Design review of the part built by this model. Coordinates are the model's own, in mm. A direction names the side the tool comes from. Give positions to 0.01 mm unless a question says otherwise; leave off trailing zeros. Order: outer loops, then holes, each group sorted by start corner. A loop starts at its lowest first (then second) coordinate and runs counter-clockwise, first axis right, second up. Notation, with made-up numbers: (16, 38.25) -> (69, 38.25) arc R13 cw to (69, 58.25) -> close; hole circle Ø3 at (45.5, -4). An arc over 180 degrees is marked (long way). One line per item, written item: value.
Autodesk Inventor part; units mm, degrees
ref_plane "Work Plane1" through (0, 0, 0) normal (0, 0.7071068, -0.7071068) x (-1, 0, 0)
ref_plane "YZ Plane" through (0, 0, 0) normal (1, 0, 0) x (0, 1, 0)
sketch "Sketch1" plane through (0, 0, 0) normal (1, 0, 0) x (0, 1, 0)
  circle A0 centre (0, 0) radius 16
  circle A1 centre (0, 13) radius 2
  circle A2 centre (0, -13) radius 2
  circle A3 centre (-13, 0) radius 2
  circle A4 centre (13, 0) radius 2
  circle A5 centre (0, -13) radius 2
  circle A6 centre (0, 13) radius 2
  circle A7 centre (13, 0) radius 2
  circle A8 centre (-13, 0) radius 2
  circle A9 centre (0, 0) radius 6.35
  line L0 (0, -22.4) -> (0, 22.4)
  dimension "d0" = 32
  dimension "d1" = 4
  dimension "d2" = 26
  dimension "d3" = 13
  dimension "d6" = 360
  dimension "d8" = 12.7
extrude "Extrusion1" add sketch "Sketch1" along normal blind 3 contours A0 L0 A2 A9 A1 | L0 A1 A9 A2 A0
sketch "Sketch2" plane through (3, 0, 0) normal (1, 0, 0) x (0, 0, -1)
  circle A0 centre (0, 0) radius 16
  circle A1 centre (13, 0) radius 2
  circle A2 centre (0, 0) radius 6.35
  circle A3 centre (0, -13) radius 2
  circle A4 centre (-13, 0) radius 2
  circle A5 centre (0, 13) radius 2
  circle A6 centre (0, 0) radius 7.5
  dimension "d11" = 15
extrude "Extrusion2" add sketch "Sketch2" along normal blind 10 contours A6
ref_plane "Work Plane1" through (0, 0, 0) normal (0, 0.7071068, -0.7071068) x (-1, 0, 0)
sketch "Sketch6" plane through (3, 0, 0) normal (1, 0, 0) x (0, 0, -1)
  circle A0 centre (0, 0) radius 7.5565
  circle A1 centre (0, 0) radius 6.35
  circle A2 centre (0, 0) radius 7.5
  circle A3 centre (0, 0) radius 6.35
  dimension "d18" = 15.113
sketch "Sketch6 outline for Extrusion4" plane through (3, 0, 0) normal (1, 0, 0) x (0, 0, -1)
  circle A0 centre (0, 0) radius 7.5565
  circle A1 centre (0, 0) radius 7.5
extrude "Extrusion4" add sketch "Sketch6 outline for Extrusion4" along normal up to surface (10 mm away)
sketch "Sketch7" plane through (3, 0, 0) normal (1, 0, 0) x (0, 0, -1)
  circle A0 centre (-13, 0) radius 2
  circle A1 centre (-13, 0) radius 3
  circle A2 centre (0, 13) radius 2
  circle A3 centre (0, 13) radius 3
  circle A4 centre (13, 0) radius 2
  circle A5 centre (13, 0) radius 2.999819
  circle A6 centre (0, -13) radius 2
  circle A7 centre (0, -13) radius 3
  circle A8 centre (0, 0) radius 7.5565
  circle A9 centre (0, 0) radius 16
  circle A10 centre (0, 13) radius 3.81
  circle A11 centre (-13, 0) radius 3.81
  circle A12 centre (0, -13) radius 3.81
  circle A13 centre (13, 0) radius 3.81
  line L0 (-13, 3.81) -> (-15.539752, 3.81)
  line L1 (-13, -3.81) -> (-15.539752, -3.81)
  line L2 (-3.81, -13) -> (-3.81, -15.539752)
  line L3 (3.81, -13) -> (3.81, -15.539752)
  line L4 (13, -3.81) -> (15.539752, -3.81)
  line L5 (13, 3.81) -> (15.539752, 3.81)
  line L6 (-3.81, 13) -> (-3.81, 15.539752)
  line L7 (3.81, 13) -> (3.81, 15.539752)
  point P0 (15.787842, -2.596928)
  point P1 (15.787842, 2.596928)
  point P2 (2.596928, 15.787842)
  point P3 (-2.596928, 15.787842)
  point P4 (-15.787842, 2.596928)
  point P5 (-15.787842, -2.596928)
  point P6 (-2.596928, -15.787842)
  point P7 (2.596928, -15.787842)
  dimension "d21" = 7.62
  dimension "d22" = 7.62
  dimension "d23" = 7.62
  dimension "d24" = 7.62
extrude "Extrusion5" add sketch "Sketch7" along normal up to surface (10 mm away) contours A1 | A9 A11 | A9 L0 A11 | A11 L1 A9 | A9 L6 A10 L7 L5 A13 L4 L3 A12 L2 L1 A11 L0 | A9 A10 L6 | L2 A12 A9 | A3 | A9 A10 | A7 | A12 A9 | A9 L7 A10 | A12 L3 A9 | A9 A13 L5 | L4 A13 A9 | A5 | A9 A13 picked at (-9.491842, -0.282602) picked at (3.503096, 12.696069) picked at (3.503096, -12.696069) picked at (12.57554, -3.495745)
sketch "Sketch8" plane through (13, 0, 0) normal (1, 0, 0) x (0, 0, -1)
  circle A0 centre (0, -13) radius 2
  circle A1 centre (-13, 0) radius 2
  line L0 (-4.495748, -4.495171) -> (-3.429275, -5.671093)
  line L1 (-4.495748, -4.495171) -> (-5.56222, -3.319249)
  circle A2 centre (0, 0) radius 6.35
  line L2 (-5.56222, -3.319249) -> (-5.465977, -3.231964)
  line L3 (-3.429275, -5.671093) -> (-3.214472, -5.476283)
  line L4 (-3.214472, -5.476283) -> (-5.45172, -3.219033)
  line L5 (-5.45172, -3.219033) -> (-6.579236, -4.336559)
  line L6 (-3.214472, -5.476283) -> (-4.341988, -6.593808)
  line L7 (-6.579236, -4.336559) -> (-4.344185, -6.591592)
  line L8 (-4.341988, -6.593808) -> (-4.344185, -6.591592)
  dimension "d27" = 1.5875
  dimension "d28" = 1.5875
  dimension "d29" = 1.5875
  dimension "d30" = 1.5875
  dimension "d31" = 90
  dimension "d32" = 0
  dimension "d33" = 90
  dimension "d34" = 3.175
  dimension "d35" = 90
extrude "Extrusion6" cut sketch "Sketch8" against normal up to surface (13 mm away) contours L1 A2 L3 L0 | L0 L3 L6 L8 L7 L5 L1 | L1 L5 A2 | A2 L5 L4 picked at (-4.633855, -4.096279)
sketch "Sketch9" plane through (13, 0, 0) normal (1, 0, 0) x (0, 0, -1)
  line L0 (-3.214472, -5.476283) -> (-4.341988, -6.593808)
  line L1 (-4.341988, -6.593808) -> (-6.579236, -4.336559)
  line L2 (-6.579236, -4.336559) -> (-5.46553, -3.232721)
  arc A0 (-3.214472, -5.476283) -> (-5.46553, -3.232721) centre (0, 0) ccw
  circle A1 centre (0, 13) radius 2
  circle A2 centre (-13, 0) radius 2
  circle A3 centre (0, -13) radius 2
  circle A4 centre (13, 0) radius 2
  circle A5 centre (0, 0) radius 16
extrude "Extrusion7" add sketch "Sketch9" along normal blind 6.0452
sketch "Sketch10" plane through (19.0452, 0, 0) normal (1, 0, 0) x (0, 0, -1)
  circle A0 centre (13, 0) radius 2
  point P0 (0, 0)
hole "Hole1" at (19.0452, 0, -13) direction (-1, 0, 0) diameter 4.4958 end through all counterbore diameter 7.62 counterbore depth 12.7
sketch "Sketch11" plane through (19.0452, 0, 0) normal (1, 0, 0) x (0, 0, -1)
  circle A0 centre (0, 13) radius 2
  point P0 (0, 0)
  point P1 (0, 13)
hole "Hole2" at (19.0452, 13, 0) direction (-1, 0, 0) diameter 4.4958 end through all counterbore diameter 7.62 counterbore depth 12.7
sketch "Sketch12" plane through (19.0452, 0, 0) normal (1, 0, 0) x (0, 0, -1)
  circle A0 centre (-13, 0) radius 2
  point P0 (0, 0)
hole "Hole3" at (19.0452, 0, 13) direction (-1, 0, 0) diameter 4.4958 end through all counterbore diameter 7.62 counterbore depth 12.7
sketch "Sketch13" plane through (19.0452, 0, 0) normal (1, 0, 0) x (0, 0, -1)
  circle A0 centre (0, -13) radius 2
  point P0 (0, 0)
  point P1 (0, -13)
hole "Hole4" at (19.0452, -13, 0) direction (-1, 0, 0) diameter 4.4958 end through all counterbore diameter 7.62 counterbore depth 12.7
properties part number "HipCoupler V2" material "Steel, Mild"
Item 1: To check wall thickness, follow line 1 along Y through (x, z) = (5.25, 0); line 2 along Y through (x, z) = (11.25, 0). State the ranges of each line that lie inside material, in increasing order. Write a range as from..to.
Returned:
line 1: -16..-15.25, -10.75..-6.35, 6.35..10.75, 15.25..16
line 2: -9.19..-6.35, 6.35..9.19
Item 2: Add section A-A on z = 12.5. Give the boundary of the cut face in (x, y).
Returned:
outline: (0, -9.99) -> (19.05, -9.99) -> (19.05, -3.78) -> (6.35, -3.78) -> (6.35, -2.19) -> (0, -2.19) -> close; (0, 2.19) -> (6.35, 2.19) -> (6.35, 3.78) -> (19.05, 3.78) -> (19.05, 9.99) -> (0, 9.99) -> close
Item 3: Clearance check with flat-ended pins moving along their axes: P1, Ø3, axis at x = 17, y = 8, coming from the +Z side; P2, Ø7.5, axis at y = 0, z = 0, coming from the -X side; P3, Ø2, axis at x = 3.5, z = 12.5, coming from the +Y side; P4, Ø5.5, axis at y = 1, z = -12, coming from the +X side. State where each tip first meets the part, or that it passes through.
Returned:
P1: z = 14.62
P2: through
P3: y = 11.12
P4: x = 19.05
Item 4: Add section C-C on y = -12. Give the boundary of the cut face in (x, z), plus the area to 3 significant figures.
Returned:
outline: (0, -10.58) -> (19.05, -10.58) -> (19.05, -3.68) -> (6.35, -3.68) -> (6.35, -2.01) -> (0, -2.01) -> close; (0, 2.01) -> (6.35, 2.01) -> (6.35, 3.68) -> (19.05, 3.68) -> (19.05, 10.58) -> (0, 10.58) -> close
area: 284 mm²
Item 5: Add section D-D on x = 4. Count the separate pieces of the cut face and the enclosed holes in it, plus the area to 4 significant figures.
Returned:
separate pieces: 1
enclosed holes: 5
area: 609.5 mm²
Item 6: Draft analysis for pull direction Z (two halves, no side actions). For faces 1 (the cylindrical face through (12.606, -0.128, -9.192)), 2 (the flat face through (0, 0, -7)), state which applies: pulls with the +Z half, pulls with the -Z half, needs draft (parallel to the pull), parting line crosses it, or undercut.
Returned:
face 1: undercut
face 2: needs draft
Item 7: Machinability: for faces 3 (the flat face through (6.345, 0, 10)), 4 (the flat face through (19.045, 7, 0)), 5 (the flat face through (9.656, -6.027, 3.77)), which of the approach directions +Z, -Z, +X, -X, +Y, -Y give a long, thin tool a straight path to every point of the face, cutting with its end or side? Answer none if there is none.
Returned:
face 3: +X
face 4: +Z, -Z, +X, +Y, -Y
face 5: +X, -X
